Can you work these out from the drawing? Everything is in mm from the part's minimum corner. A direction names the side the tool comes from. Coordinates: 2 decimals unless noted, no trailing zeros. Loops run counter-clockwise (first coordinate to the right, second up) from the corner with the lowest first, then second, coordinate; pieces in that order, holes last. Notation, with made-up numbers: (-10, 62) - (14, 62) arc R26 cw to (14, 83) - close; hole circle Ø5 at (-6.75, 13). An arc over 180 degrees is marked (long way). One line per question, with ' | ' between items. Start each with the question number.
1. Which directions (+Z, -Z, +X, -X, +Y, -Y) give clear straight access to the entire face, cutting with the end or side of a thin tool? Please do the marked faces 5, 6 and 7.
2. I want a section at B-B, the plane y = 2.5. Write out the boundary of the cut face in (x, z).
3. I want a section at C-C, the plane x = 5. Write out the boundary of the cut face in (y, z).
4. I want a section at A-A, the plane z = 10. Write out the boundary of the cut face in (x, y), then the cut area to 3 significant figures.
5. I'm going to push flat-ended pins straight in: P1, Ø2, axis at y = 2, z = 34.5, coming from the +X side; P2, Ø4, axis at x = 8.5, y = 8.5, coming from the -Z side; P3, Ø6, axis at x = 8, z = 50, coming from the +Y side; P4, Ø2, axis at x = 4, y = 5.5, coming from the +Z side. Where does each tip first touch, or does it pass through?
6. I want a section at D-D, the plane x = 2. Write out the boundary of the cut face in (y, z), then the cut area to 3 significant figures.
7. Please list where these lines run through material, in increasing order: L1, parallel to Z at x = 7.5, y = 2.75; L2, parallel to X at y = 0.4, z = 10; L3, parallel to Y at x = 3.25, z = 2.5. Write a range as [from, to].
8. We'd pull the mould along Z, two halves only. Please class the marked faces 1, 2, 3 and 4: pulls with the +Z half, pulls with the -Z half, needs draft (parallel to the pull), parting line crosses it, or undercut.
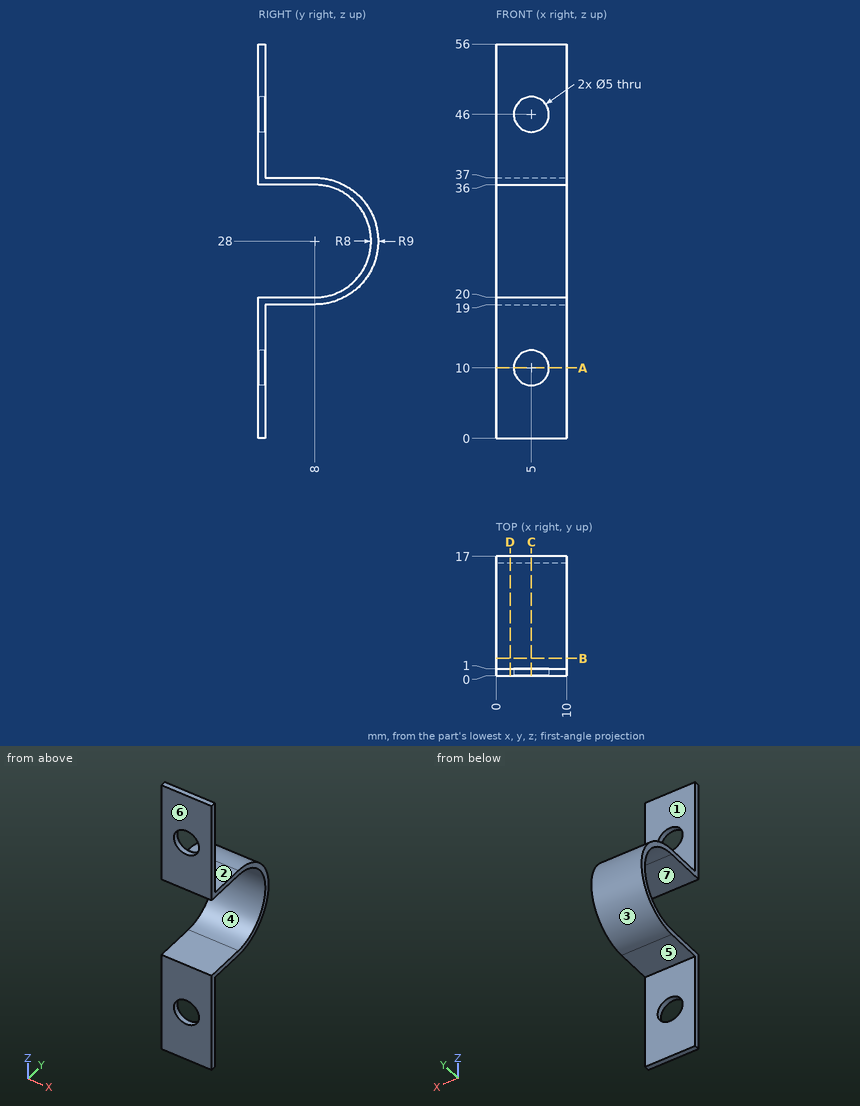
Results are:
1) face 5: -Z, +X, -X, +Y | face 6: +Z, -Z, +X, -X, -Y | face 7: +X, -X, -Y
2) outline: (0, 19) - (10, 19) - (10, 20) - (0, 20) - close; (0, 36) - (10, 36) - (10, 37) - (0, 37) - close
3) outline: (0, 0) - (1, 0) - (1, 7.5) - (0, 7.5) - close; (0, 12.5) - (1, 12.5) - (1, 19) - (8, 19) arc R9 ccw to (8, 37) - (1, 37) - (1, 43.5) - (0, 43.5) - (0, 36) - (8, 36) arc R8 cw to (8, 20) - (0, 20) - close; (0, 48.5) - (1, 48.5) - (1, 56) - (0, 56) - close
4) outline: (0, 0) - (2.5, 0) - (2.5, 1) - (0, 1) - close; (7.5, 0) - (10, 0) - (10, 1) - (7.5, 1) - close | area: 5.00 mm2
5) P1: passes through | P2: stops at z = 19 | P3: stops at y = 1 | P4: stops at z = 37
6) outline: (0, 0) - (1, 0) - (1, 19) - (8, 19) arc R9 ccw to (8, 37) - (1, 37) - (1, 56) - (0, 56) - (0, 36) - (8, 36) arc R8 cw to (8, 20) - (0, 20) - close | area: 80.7 mm2
7) L1: z = [19, 20], [36, 37] | L2: x = [0, 2.5], [7.5, 10] | L3: y = [0, 1]
8) face 1: needs draft | face 2: pulls with the +Z half | face 3: parting line crosses it | face 4: undercut
